CAD build for the part. Positions are in the model's coordinates, mm. Face numbers are marked on the shaded views. A direction names the side the tool comes from. Round coordinates to 2 decimals unless told otherwise and drop trailing zeros. Write each loop counter-clockwise with the first axis right and the second up, starting at its lowest first coordinate (ties: lowest second). Pieces come first, ordered by that corner, then holes. Notation, with made-up numbers: (28, 17) - (60, 17) arc R16 ccw to (60, 43) - close; hole circle Ø4 at (25, 16). An arc over 180 degrees is marked (long way). Answer in a Markdown table with one row per item.
```python
from build123d import *

# Parameters (mm, degrees)
SKETCH1_W                        = 46
SKETCH1_H                        = 46
BOSS_EXTRUDE1_DEPTH              = 2.5
SKETCH2_W                        = 46
SKETCH2_H                        = 48.5
BOSS_EXTRUDE2_DEPTH              = 2.5
SKETCH3_W                        = 56
SKETCH3_H                        = 51
BOSS_EXTRUDE3_DEPTH              = 2.5
SKETCH7_W                        = 5
SKETCH7_H                        = 10
BOSS_EXTRUDE6_DEPTH              = 15
CBORE_FOR_M2_5_SHCS1_D           = 3.1
CBORE_FOR_M2_5_SHCS1_DEPTH       = 5
CBORE_FOR_M2_5_SHCS1_CBORE_D     = 5.5
CBORE_FOR_M2_5_SHCS1_CBORE_DEPTH = 3.5
CBORE_FOR_M2_5_SHCS1_TIP         = 0.931333959
SKETCH11_W                       = 19
SKETCH11_H                       = 19
CUT_EXTRUDE2_DEPTH               = 71.299359883
M3X0_5_TAPPED_HOLE1_D            = 2.5
FILLET1_R                        = 3
MOVE_FACE1_BY                    = 0.1
MOVE_FACE1_2_BY                  = 0.1
MOVE_FACE1_3_BY                  = 0.1
MOVE_FACE1_4_BY                  = 0.1
MOVE_FACE2_BY                    = 0.1
MOVE_FACE2_2_BY                  = 0.1
M2_5X0_45_TAPPED_HOLE1_D         = 2.05
M2_5X0_45_TAPPED_HOLE1_DEPTH     = 5
M2_5X0_45_TAPPED_HOLE1_TIP       = 0.615882135
CBORE_FOR_M2_5_SHCS2_D           = 3.1
CBORE_FOR_M2_5_SHCS2_DEPTH       = 5
CBORE_FOR_M2_5_SHCS2_CBORE_D     = 5.5
CBORE_FOR_M2_5_SHCS2_CBORE_DEPTH = 3.5
CBORE_FOR_M2_5_SHCS2_TIP         = 0.931333959


with BuildPart() as part:
    # Sketch1 → Boss-Extrude1 (new body)
    with BuildSketch(Plane(origin=(0, 0, 0), x_dir=(1, 0, 0), z_dir=(0, 1, 0))):
        with Locations((23, 23)):
            Rectangle(SKETCH1_W, SKETCH1_H)
    extrude(amount=BOSS_EXTRUDE1_DEPTH)

    # Sketch2 → Boss-Extrude2 (add)
    with BuildSketch(Plane(origin=(0, 2.5, 0), x_dir=(1, 0, 0), z_dir=(0, 1, 0))):
        with Locations((23, 21.75)):
            Rectangle(SKETCH2_W, SKETCH2_H)
    extrude(amount=BOSS_EXTRUDE2_DEPTH)

    # Sketch3 → Boss-Extrude3 (add)
    with BuildSketch(Plane.XZ):
        with Locations((23, -20.5)):
            Rectangle(SKETCH3_W, SKETCH3_H)
    extrude(amount=BOSS_EXTRUDE3_DEPTH)

    # Sketch7 → Boss-Extrude6 (add)
    with BuildSketch(Plane.XZ.offset(2.5)):
        with Locations((11, -20.5)):
            Rectangle(SKETCH7_W, SKETCH7_H)
        with Locations((35, -20.5)):
            Rectangle(SKETCH7_W, SKETCH7_H)
    extrude(amount=BOSS_EXTRUDE6_DEPTH)

    # CBORE for M2.5 SHCS1
    with Locations(Plane.ZY.offset(-8.5)):
        with Locations((-20.5, -10.5)):
            CounterBoreHole(CBORE_FOR_M2_5_SHCS1_D / 2, CBORE_FOR_M2_5_SHCS1_CBORE_D / 2, CBORE_FOR_M2_5_SHCS1_CBORE_DEPTH, depth=CBORE_FOR_M2_5_SHCS1_DEPTH)
            with Locations((0, 0, -(CBORE_FOR_M2_5_SHCS1_DEPTH + CBORE_FOR_M2_5_SHCS1_TIP / 2))):  # 118° drill point
                Cone(0, CBORE_FOR_M2_5_SHCS1_D / 2, CBORE_FOR_M2_5_SHCS1_TIP, mode=Mode.SUBTRACT)

    # Sketch11 → Cut-Extrude2 (cut, through all)
    with BuildSketch(Plane.XZ.offset(2.5)):
        with Locations((23, -20.5)):
            Rectangle(SKETCH11_W, SKETCH11_H)
    extrude(amount=-CUT_EXTRUDE2_DEPTH, mode=Mode.SUBTRACT)

    # M3x0.5 Tapped Hole1 (through all)
    with Locations(Plane(origin=(0, 5, 0), x_dir=(1, 0, 0), z_dir=(0, 1, 0))):
        with Locations((5.5, 38), (40.5, 38), (40.5, 3), (5.5, 3)):
            Hole(M3X0_5_TAPPED_HOLE1_D / 2)

    # Fillet1
    fillet1_edges = [part.edges().sort_by_distance(p)[0] for p in [
        (51, -1.25, 5),
        (-5, -1.25, 5),
    ]]
    fillet(fillet1_edges, radius=FILLET1_R)

    # Move Face1: a face moved inward by 0.1
    extrude(part.faces().sort_by_distance((23, 5, -9.625))[0], amount=MOVE_FACE1_BY, dir=(0, -1, 0), mode=Mode.SUBTRACT)

    # Move Face1 2: a face moved inward by 0.1
    extrude(part.faces().sort_by_distance((23, 2.5, 1.25))[0], amount=MOVE_FACE1_2_BY, dir=(0, 1, 0), mode=Mode.SUBTRACT)

    # Move Face1 3: a face moved inward by 0.1
    extrude(part.faces().sort_by_distance((23, 3.75, 2.5))[0], amount=MOVE_FACE1_3_BY, dir=(0, 0, -1), mode=Mode.SUBTRACT)

    # Move Face1 4: a face moved inward by 0.1
    extrude(part.faces().sort_by_distance((23, 1.25, 0))[0], amount=MOVE_FACE1_4_BY, dir=(0, 0, -1), mode=Mode.SUBTRACT)

    # Move Face2: a face moved inward by 0.1
    extrude(part.faces().sort_by_distance((0, 2.482407006, -22.446731119))[0], amount=MOVE_FACE2_BY, dir=(1, 0, 0), mode=Mode.SUBTRACT)

    # Move Face2 2: a face moved inward by 0.1
    extrude(part.faces().sort_by_distance((46, 2.482407006, -22.446731119))[0], amount=MOVE_FACE2_2_BY, dir=(-1, 0, 0), mode=Mode.SUBTRACT)

    # M2.5x0.45 Tapped Hole1
    with Locations(Plane(origin=(0, 0, -46), x_dir=(-1, 0, 0), z_dir=(0, 0, -1))):
        with Locations((-36, 1.9), (-10, 1.9)):
            Hole(M2_5X0_45_TAPPED_HOLE1_D / 2, depth=M2_5X0_45_TAPPED_HOLE1_DEPTH)
            with Locations((0, 0, -(M2_5X0_45_TAPPED_HOLE1_DEPTH + M2_5X0_45_TAPPED_HOLE1_TIP / 2))):  # 118° drill point
                Cone(0, M2_5X0_45_TAPPED_HOLE1_D / 2, M2_5X0_45_TAPPED_HOLE1_TIP, mode=Mode.SUBTRACT)

    # CBORE for M2.5 SHCS2
    with Locations(Plane(origin=(37.5, 0, 0), x_dir=(0, 0, -1), z_dir=(1, 0, 0))):
        with Locations((20.5, -10.5)):
            CounterBoreHole(CBORE_FOR_M2_5_SHCS2_D / 2, CBORE_FOR_M2_5_SHCS2_CBORE_D / 2, CBORE_FOR_M2_5_SHCS2_CBORE_DEPTH, depth=CBORE_FOR_M2_5_SHCS2_DEPTH)
            with Locations((0, 0, -(CBORE_FOR_M2_5_SHCS2_DEPTH + CBORE_FOR_M2_5_SHCS2_TIP / 2))):  # 118° drill point
                Cone(0, CBORE_FOR_M2_5_SHCS2_D / 2, CBORE_FOR_M2_5_SHCS2_TIP, mode=Mode.SUBTRACT)


solid = part.part
```
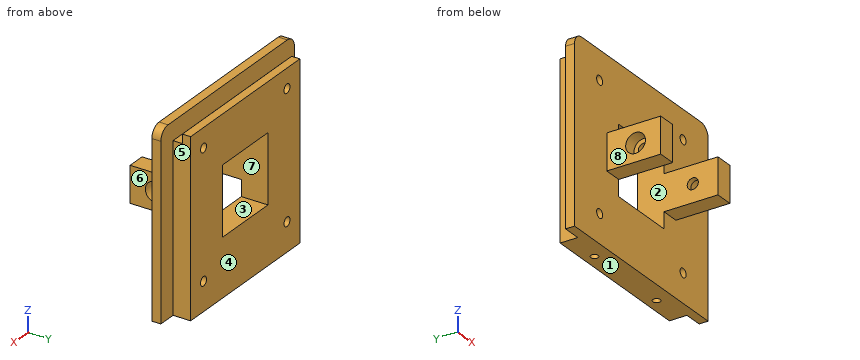
Q1. Pull direction Z, two halves, no side cores. Call the marked faces 1, 2, 3 and 4: released by +Z, released by -Z, zero draft, split by the parting line, or undercut.
Computed:
| item | result |
|---|---|
| face 1 | released by -Z |
| face 2 | undercut |
| face 3 | undercut |
| face 4 | zero draft |
Q2. Drill centre lines: line 1 (X direction, y = 1.75, z = -38); line 2 (Z direction, x = 20.5, y = -0.25); line 3 (X direction, y = 1.9, z = -44.1) (3 decimals). Where is each one in solid material? Low to high.
Computed:
| item | result |
|---|---|
| line 1 | x = 0.1 to 4.25, 6.75 to 39.25, 41.75 to 45.9 |
| line 2 | z = -46 to -30, -11 to 5 |
| line 3 | x = 0.1 to 8.975, 11.025 to 34.975, 37.025 to 45.9 |
Q3. Saw through at A-A on x = 5.5. List the corners of the cut face in (y, z), then the cut area to 3 significant figures.
Computed:
| item | result |
|---|---|
| outline | (-2.5, -46) - (4.9, -46) - (4.9, -39.25) - (-2.5, -39.25) - close; (-2.5, -36.75) - (4.9, -36.75) - (4.9, -4.25) - (-2.5, -4.25) - close; (-2.5, -1.75) - (4.9, -1.75) - (4.9, 2.4) - (2.6, 2.4) - (2.6, -0.1) - (0, -0.1) - (0, 5) - (-2.5, 5) - close |
| area | 321 mm2 |
Q4. Saw through at D-D on z = -3. List the corners of the cut face in (x, y).
Computed:
| item | result |
|---|---|
| outline | (-5, -2.5) - (4.25, -2.5) - (4.25, 4.9) - (0.1, 4.9) - (0.1, 0) - (-5, 0) - close; (6.75, -2.5) - (39.25, -2.5) - (39.25, 4.9) - (6.75, 4.9) - close; (41.75, -2.5) - (51, -2.5) - (51, 0) - (45.9, 0) - (45.9, 4.9) - (41.75, 4.9) - close |
Q5. 3-axis set-ups, long thin cutter, end or side, ignore diameter. For the marked faces 5, 6, 7 and 8: which of +Z, -Z, +X, -X, +Y, -Y reach the whole face in a straight line?
Computed:
| item | result |
|---|---|
| face 5 | +Z, -Z, +X, +Y |
| face 6 | +Z, -Z, +X, -Y |
| face 7 | +Y, -Y |
| face 8 | +Z, -Z, -X, -Y |
Q6. Saw through at C-C on y = 3.75. List the corners of the cut face in (x, z), then the cut area to 3 significant figures.
Computed:
| item | result |
|---|---|
| outline | (0.1, -46) - (45.9, -46) - (45.9, 2.4) - (0.1, 2.4) - close; hole circle Ø2.5 at (5.5, -38); hole circle Ø2.5 at (5.5, -3); hole (13.5, -30) - (32.5, -30) - (32.5, -11) - (13.5, -11) - close; hole circle Ø2.5 at (40.5, -38); hole circle Ø2.5 at (40.5, -3) |
| area | 1,840 mm2 |
Q7. Saw through at B-B on z = -20.5. Count the separate pieces of the cut face and the enclosed holes in it, then the cut area to 3 significant figures.
Computed:
| item | result |
|---|---|
| separate pieces | 4 |
| enclosed holes | 0 |
| area | 326 mm2 |
Q8. Flat gauge pins, fed straight in: pin 1 (4 mm diameter, centred on y = 3, z = -20, fed in from +X); pin 2 (5 mm diameter, centred on y = -10.5, z = -20.5, fed in from +X); pin 3 (5.5 mm diameter, centred on x = 36, y = -13, fed in from +Z). Where does each tip first touch, or does it go through?
Computed:
| item | result |
|---|---|
| pin 1 | stops at x = 45.9 |
| pin 2 | stops at x = 34 |
| pin 3 | stops at z = -15.5 |
